from build123d import *

# Parameters (mm, degrees)
F1_W        = 17.5
F1_H        = 17.5
F1_W_2      = 13.5
F1_H_2      = 13.5
F2_DEPTH    = 25
F3_W        = 17.5
F3_H        = 17.5
F3_W_2      = 13.5
F3_H_2      = 13.5
F4_DEPTH    = 25
F6_DEPTH    = 17.5
F7_T1_DEPTH = 18.2385988642
F7_T3_DEPTH = 27.8540843944
F7_T5_DEPTH = 27.867199163
F8_R        = 15


# Not quite as in the source:
# - a fillet or chamfer that OpenCascade refuses, or shapes differently, is made with other operations: its cross-section is extruded or revolved along the edge and cut away or added


with BuildPart() as f2:
    # F1 (on Top) → F2 (new body)
    with BuildSketch(Plane.XY):
        Rectangle(F1_W, F1_H)
        Rectangle(F1_W_2, F1_H_2, mode=Mode.SUBTRACT)
    extrude(amount=F2_DEPTH)

    # F3 (on face) → F4 (join)
    with BuildSketch(Plane(origin=(0, 8.75, 0), x_dir=(-1, 0, 0), z_dir=(0, 1, 0))):
        with Locations((0, -8.75)):
            Rectangle(F3_W, F3_H)
        with Locations((0, -8.75)):
            Rectangle(F3_W_2, F3_H_2, mode=Mode.SUBTRACT)
    extrude(amount=F4_DEPTH)

    # F5 (on face) → F6 (join, through all)
    with BuildSketch(Plane(origin=(-8.75, 0, 0), x_dir=(0, -1, 0), z_dir=(-1, 0, 0))):
        Polygon((-8.75, 0), (-8.75, -17.5), (8.7529988959, 0), align=None)
    extrude(amount=-F6_DEPTH)

    # F7: fillet of radius 5 on 3 edges, made by hand

    # F7_s2 → F7_t1 (cut)
    with BuildSketch(Plane.YZ.offset(-9.1192994321)):
        with BuildLine():
            ThreePointArc((-8.75, 0), (-8.6996483838, -0.052591736), (-8.6485362941, -0.1044447036))
            Line((-8.6485362941, -0.1044447036), (-8.7529988959, 0))
            Line((-8.7529988959, 0), (-8.75, 0))
        make_face()
    extrude(amount=F7_T1_DEPTH, mode=Mode.SUBTRACT)

    # F7_s4 → F7_t3 (cut)
    with BuildSketch(Plane.YZ.offset(-13.9270421972)):
        with BuildLine():
            ThreePointArc((7.2855858942, -16.0358368012), (8.9075976032, -17.1194796247), (10.8208168789, -17.5))
            Line((10.8208168789, -17.5), (8.75, -17.5))
            Line((8.75, -17.5), (7.2855858942, -16.0358368012))
        make_face()
    extrude(amount=F7_T3_DEPTH, mode=Mode.SUBTRACT)

    # F7_s6 → F7_t5 (cut)
    with BuildSketch(Plane.YZ.offset(-13.9335995815)):
        with BuildLine():
            ThreePointArc((-8.75, 2.0683203716), (-8.3693156919, 0.1547053272), (-7.2852309847, -1.4675164296))
            Line((-7.2852309847, -1.4675164296), (-7.6387540831, -1.8211001097))
            ThreePointArc((-7.6387540831, -1.8211001097), (-9.0020593926, -0.4580283837), (-9.1136694691, -0.3431392098))
            Line((-9.1136694691, -0.3431392098), (-9.25, 0))
            Line((-9.25, 0), (-9.25, 2.0683203716))
            Line((-9.25, 2.0683203716), (-8.75, 2.0683203716))
        make_face()
    extrude(amount=F7_T5_DEPTH, mode=Mode.SUBTRACT)

    # F8
    f8_edges = [f2.edges().sort_by_distance(p)[0] for p in [
        (0, 8.75, 0),
    ]]
    fillet(f8_edges, radius=F8_R)


solid = f2.part
Geometry check sheet. Reference: the model listing, model coordinates, mm. A direction names the side the tool comes from. Round coordinates to 2 decimals unless told otherwise and drop trailing zeros. Loops run counter-clockwise (first coordinate to the right, second up) from the corner with the lowest first, then second, coordinate; pieces in that order, holes last. Notation, with made-up numbers: (89.5, 78) - (137.5, 78) arc R31 cw to (137.5, 110) - close; hole circle Ø9 at (35, -27). An arc over 180 degrees is marked (long way). One line per question, with ' | ' between items. Start each with the question number.
1. Cross-section at C-C on z = 16. Record the cut outline in (x, y).
2. Cross-section at D-D on y = -0.5. Record the cut outline in (x, z), then the cut area to 3 significant figures.
3. Cross-section at B-B on x = -3. Record the cut outline in (y, z).
4. Cross-section at A-A on y = 25.5. Record the cut outline in (x, z).
5. Draft check along X on faces 1 (the face through (0, 0, 0)), 2 (the face through (-8.75, 7, -1)), 3 (the face through (0.12, 13.26, 4.28)). Enter one of: released by +X, released by -X, zero draft, split by the parting line, or undercut.
6. Depth check by flat-ended pin: pin 1 (4 mm diameter, centred on x = 0.5, z = 11, fed in from +Y); pin 2 (2 mm diameter, centred on x = 6, z = 16.5, fed in from +Y); pin 3 (8 mm diameter, centred on x = 2.5, z = 17.5, fed in from +Y). Enter the tip coordinate at first touch or a pass-through.
7. Tool access check on faces 4 (the face through (0, 21, -15.5)), 5 (the face through (0, 22, -17.5)), 6 (the face through (0, 29, 0)), 7 (the face through (0, -6.75, 12)). Record the directions out of +Z, -Z, +X, -X, +Y, -Y that give a thin tool (end or side, any length) a straight path to the whole face; none if there is none.
8. Scan lines: line 1 (Z direction, x = 2.75, y = 23.5); line 2 (X direction, y = 0, z = 15.5). Record each from-to range of solid material in increasing order. Write a range as [from, to].
Taken from the geometry:
1) outline: (-8.75, -8.75) - (8.75, -8.75) - (8.75, 8.75) - (-8.75, 8.75) - close; hole (-6.75, -6.75) - (6.75, -6.75) - (6.75, 6.75) - (-6.75, 6.75) - close
2) outline: (-8.75, -8.25) - (8.75, -8.25) - (8.75, 25) - (6.75, 25) - (6.75, 0) - (-6.75, 0) - (-6.75, 25) - (-8.75, 25) - close | area: 244 mm²
3) outline: (-8.75, 2.07) arc R5 ccw to (-7.29, -1.47) - (7.29, -16.04) arc R5 ccw to (10.82, -17.5) - (33.75, -17.5) - (33.75, -15.5) - (8.75, -15.5) - (8.75, -2) - (33.75, -2) - (33.75, 0) - (23.75, 0) arc R15 cw to (8.75, 15) - (8.75, 25) - (6.75, 25) - (6.75, 0) - (-6.75, 0) - (-6.75, 25) - (-8.75, 25) - close
4) outline: (-8.75, -17.5) - (8.75, -17.5) - (8.75, 0) - (-8.75, 0) - close; hole (-6.75, -15.5) - (6.75, -15.5) - (6.75, -2) - (-6.75, -2) - close
5) face 1: undercut | face 2: released by -X | face 3: zero draft
6) pin 1: y = 10 | pin 2: y = 8.75 | pin 3: y = 8.83
7) face 4: +Y | face 5: -Z, +X, -X, +Y, -Y | face 6: +Z, +X, -X, +Y | face 7: +Z
8) line 1: [-17.5, -15.5], [-2, 0] | line 2: [-8.75, -6.75], [6.75, 8.75]
